```python
from build123d import *

# Parameters (mm, degrees)
BOSS_EXTRUDE1_DEPTH = 5
BOSS_EXTRUDE2_DEPTH = 5
FILLET1_R           = 5
SKETCH3_R           = 5.5
SKETCH3_R_2         = 2.15
BOSS_EXTRUDE3_DEPTH = 8
SKETCH4_R           = 2.15
CUT_EXTRUDE1_DEPTH  = 6


with BuildPart() as part:
    # Sketch1 → Boss-Extrude1 (new body)
    with BuildSketch(Plane.XY):
        with BuildLine():
            Line((-44.560511167, 40.967802535), (-33.210007488, 33.020094297))
            Line((-33.210007488, 33.020094297), (14.586986289, 55.308198532))
            Line((14.586986289, 55.308198532), (11.410228171, 56.535093153))
            ThreePointArc((11.410228171, 56.535093153), (6.297014824, 63.726834744), (10.911476341, 71.248326799))
            Line((10.911476341, 71.248326799), (-52.530068751, 41.665048477))
            ThreePointArc((-52.530068751, 41.665048477), (-48.451876715, 42.384143766), (-44.560511167, 40.967802535))
        make_face()
        with BuildLine():
            Line((14.586986289, 55.308198532), (137.080557575, 8))
            Line((137.080557575, 8), (180, 8))
            ThreePointArc((180, 8), (181.465917665, 7.864546103), (182.882194265, 7.46277135))
            Line((182.882194265, 7.46277135), (17.1746167, 71.460635853))
            ThreePointArc((17.1746167, 71.460635853), (22.287830046, 64.268894262), (17.673368529, 56.747402207))
            Line((17.673368529, 56.747402207), (14.586986289, 55.308198532))
        make_face()
        with BuildLine():
            Line((137.080557575, 8), (2.522390311, 8))
            Line((2.522390311, 8), (4.588611491, 6.553216354))
            ThreePointArc((4.588611491, 6.553216354), (7.629735606, -2.405646396), (0, -8))
            Line((0, -8), (180, -8))
            ThreePointArc((180, -8), (178.534082335, -7.864546103), (177.117805735, -7.46277135))
            Line((177.117805735, -7.46277135), (137.080557575, 8))
        make_face()
        with BuildLine():
            ThreePointArc((-4.588611491, -6.553216354), (-7.629735606, 2.405646396), (0, 8))
            Line((0, 8), (2.522390311, 8))
            Line((2.522390311, 8), (-33.210007488, 33.020094297))
            Line((-33.210007488, 33.020094297), (-45.768176563, 27.164123885))
            ThreePointArc((-45.768176563, 27.164123885), (-49.846368599, 26.445028596), (-53.737734148, 27.861369827))
            Line((-53.737734148, 27.861369827), (-4.588611491, -6.553216354))
        make_face()
        with BuildLine():
            Line((180, 8), (137.080557575, 8))
            Line((137.080557575, 8), (177.117805735, -7.46277135))
            ThreePointArc((177.117805735, -7.46277135), (178.534082335, -7.864546103), (180, -8))
            ThreePointArc((180, -8), (187.864546103, -1.465917665), (182.882194265, 7.46277135))
            ThreePointArc((182.882194265, 7.46277135), (181.465917665, 7.864546103), (180, 8))
        make_face()
        with BuildLine():
            Line((11.410228171, 56.535093153), (14.586986289, 55.308198532))
            Line((14.586986289, 55.308198532), (17.673368529, 56.747402207))
            ThreePointArc((17.673368529, 56.747402207), (22.287830046, 64.268894262), (17.1746167, 71.460635853))
            ThreePointArc((17.1746167, 71.460635853), (14.021392676, 71.993272114), (10.911476341, 71.248326799))
            ThreePointArc((10.911476341, 71.248326799), (6.297014824, 63.726834744), (11.410228171, 56.535093153))
        make_face()
        with BuildLine():
            Line((-45.768176563, 27.164123885), (-33.210007488, 33.020094297))
            Line((-33.210007488, 33.020094297), (-44.560511167, 40.967802535))
            ThreePointArc((-44.560511167, 40.967802535), (-48.451876715, 42.384143766), (-52.530068751, 41.665048477))
            ThreePointArc((-52.530068751, 41.665048477), (-57.118680242, 35.111832123), (-53.737734148, 27.861369827))
            ThreePointArc((-53.737734148, 27.861369827), (-49.846368599, 26.445028596), (-45.768176563, 27.164123885))
        make_face()
        with BuildLine():
            Line((2.522390311, 8), (0, 8))
            ThreePointArc((0, 8), (-7.629735606, 2.405646396), (-4.588611491, -6.553216354))
            ThreePointArc((-4.588611491, -6.553216354), (-2.405646396, -7.629735606), (0, -8))
            ThreePointArc((0, -8), (7.629735606, -2.405646396), (4.588611491, 6.553216354))
            Line((4.588611491, 6.553216354), (2.522390311, 8))
        make_face()
    extrude(amount=BOSS_EXTRUDE1_DEPTH)

    # Sketch2 → Boss-Extrude2 (add, through all)
    with BuildSketch(Plane.XY.offset(5)):
        Polygon((14.586986289, 55.308198532), (6.740403892, 51.64927707), (31.941325759, 8), (49.261833834, 8), (24.060911968, 51.64927707), align=None)
    extrude(amount=-BOSS_EXTRUDE2_DEPTH)

    # Fillet1
    fillet1_edges = [part.edges().sort_by_distance(p)[0] for p in [
        (-33.210007488, 33.020094297, 2.5),
        (2.522390311, 8, 2.5),
        (137.080557575, 8, 2.5),
        (24.060911968, 51.64927707, 2.5),
        (49.261833834, 8, 2.5),
        (31.941325759, 8, 2.5),
        (6.740403892, 51.64927707, 2.5),
    ]]
    fillet(fillet1_edges, radius=FILLET1_R)

    # Sketch3 → Boss-Extrude3 (add)
    with BuildSketch(Plane.XY.offset(5)):
        with Locations((-49.149122657, 34.414586181)):
            Circle(SKETCH3_R)
        with Locations((-49.149122657, 34.414586181)):
            Circle(SKETCH3_R_2, mode=Mode.SUBTRACT)
        with Locations((3.981659537, 1.5)):
            Circle(SKETCH3_R)
        with Locations((3.981659537, 1.5)):
            Circle(SKETCH3_R_2, mode=Mode.SUBTRACT)
        with Locations((59.781659537, 1.5)):
            Circle(SKETCH3_R)
        with Locations((59.781659537, 1.5)):
            Circle(SKETCH3_R_2, mode=Mode.SUBTRACT)
        with Locations((114.981659537, 1.5)):
            Circle(SKETCH3_R)
        with Locations((114.981659537, 1.5)):
            Circle(SKETCH3_R_2, mode=Mode.SUBTRACT)
        with Locations((170.981659537, 1.5)):
            Circle(SKETCH3_R)
        with Locations((170.981659537, 1.5)):
            Circle(SKETCH3_R_2, mode=Mode.SUBTRACT)
        with Locations((3.45920938, 60)):
            Circle(SKETCH3_R)
        with Locations((3.45920938, 60)):
            Circle(SKETCH3_R_2, mode=Mode.SUBTRACT)
    extrude(amount=BOSS_EXTRUDE3_DEPTH)

    # Sketch4 → Cut-Extrude1 (cut, through all)
    with BuildSketch(Plane.XY.offset(5)):
        with Locations((-49.149122657, 34.414586181)):
            Circle(SKETCH4_R)
        with Locations((3.981659537, 1.5)):
            Circle(SKETCH4_R)
        with Locations((59.781659537, 1.5)):
            Circle(SKETCH4_R)
        with Locations((114.981659537, 1.5)):
            Circle(SKETCH4_R)
        with Locations((170.981659537, 1.5)):
            Circle(SKETCH4_R)
        with Locations((3.45920938, 60)):
            Circle(SKETCH4_R)
    extrude(amount=-CUT_EXTRUDE1_DEPTH, mode=Mode.SUBTRACT)


solid = part.part
```
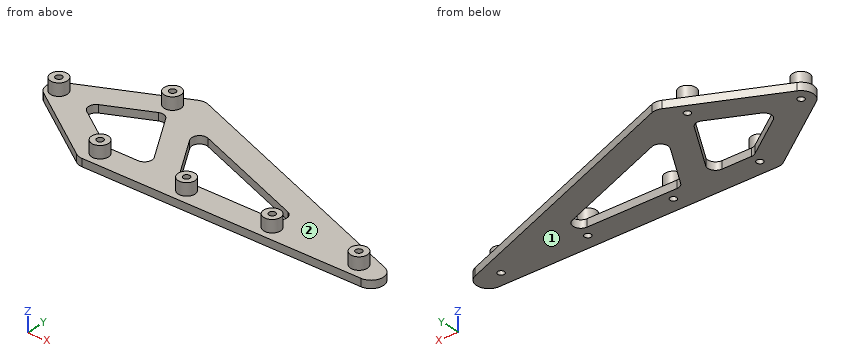
The listing builds one solid part. Answer for the finished solid, in the listing's coordinates (mm). Face numbers are marked on the shaded views. Give positions to 0.01 mm unless a question says otherwise; leave off trailing zeros. Write each loop counter-clockwise with the first axis right and the second up, starting at its lowest first coordinate (ties: lowest second). Pieces come first, ordered by that corner, then holes. Notation, with made-up numbers: M 31.25,80.25 L 36.25,80.25 A13 cw 36.25,96.25 Z; hole C 60,61.5 d2. An arc over 180 degrees is marked long. Write each question's results on one line, items separated by ' | '.
Q1. Section D-D, the plane y = 20.5 is taken. Write down the section's boundary in (x, z), then the cut area to 3 significant figures.
Output values:
outline: M -43.22,0 L -15.33,0 L -15.33,5 L -43.22,5 Z; M 24.72,0 L 42.04,0 L 42.04,5 L 24.72,5 Z; M 104.71,0 L 149.13,0 L 149.13,5 L 104.71,5 Z | area: 448 mm2
Q2. Consider L1, parallel to Z at x = 4.5, y = 50.5; L2, parallel to X at y = 34, z = 12.75; L3, parallel to Y at x = -14, z = 2.25. Determine where each line is inside the solid, lowest interval first. Write a range as from..to.
Output values:
L1: 0..5 | L2: -54.63..-51.26, -47.04..-43.66 | L3: 0.04..19.57, 41.98..59.63
Q3. Section B-B, the plane z = 7 is taken. Count the separate pieces of the cut face and the enclosed holes in it, then the cut area to 3 significant figures.
Output values:
separate pieces: 6 | enclosed holes: 6 | area: 483 mm2
Q4. Flat-ended cylindrical pins translate along their axes: P1, Ø4, axis at x = 170.98, y = 1.5, coming from the -Z side; P2, Ø1, axis at y = 63, z = 7.5, coming from the +X side; P3, Ø4, axis at x = 94, z = 1.5, coming from the +Y side; P4, Ø3, axis at x = -3, z = 1.5, coming from the +Y side. Find the tip coordinate at first contact, or state that the pin passes through.
Output values:
P1: through | P2: x = 8.36 | P3: y = 42.56 | P4: y = 65.46
Q5. Section C-C, the plane x = -18 is taken. Write down the section's boundary in (y, z), then the cut area to 3 significant figures.
Output values:
outline: M 2.84,0 L 22.37,0 L 22.37,5 L 2.84,5 Z; M 40.11,0 L 57.77,0 L 57.77,5 L 40.11,5 Z | area: 186 mm2
Q6. Section A-A, the plane y = 60 is taken. Write down the section's boundary in (x, z).
Output values:
outline: M -13.21,0 L 1.31,0 L 1.31,13 L -2.04,13 L -2.04,5 L -13.21,5 Z; M 5.61,0 L 46.85,0 L 46.85,5 L 8.96,5 L 8.96,13 L 5.61,13 Z
Q7. For a pull along X with two mould halves and no side action, classify the marked faces 1 and 2 as released by +X, released by -X, zero draft, split by the parting line, or undercut.
Output values:
face 1: zero draft | face 2: undercut
